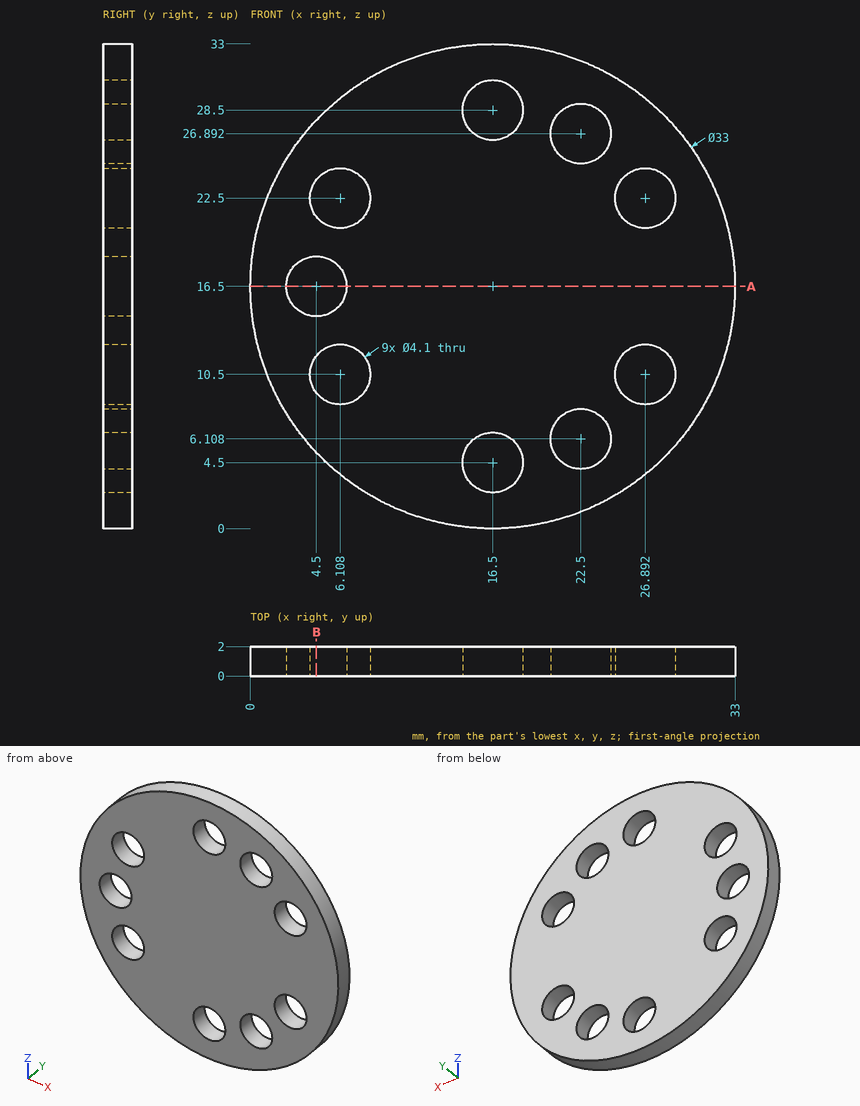
Geometry check sheet. Reference: drawing and pictorial views, mm from the part's lowest x, y, z. Round coordinates to 2 decimals unless told otherwise and drop trailing zeros. Order: outer loops, then holes, each group sorted by start corner. A loop starts at its lowest first (then second) coordinate and runs counter-clockwise, first axis right, second up. Notation, with made-up numbers: (13, 63.5) - (68, 63.5) arc R6 ccw to (68, 67.5) - close; hole circle Ø7 at (74, 49). An arc over 180 degrees is marked (long way). One line per question, with ' | ' between items. Start each with the question number.
(1) Sectioned sample at A-A on z = 16.5. Record the cut outline in (x, y).
(2) Sectioned sample at B-B on x = 4.5. Count the separate pieces of the cut face and the enclosed holes in it, and give its area (3 significant figures).
(3) Thickness scan on L1, parallel to X at y = 1.05, z = 16.5; L2, parallel to X at y = 1.2, z = 10 (1 decimal); L3, parallel to X at y = 0.8, z = 22.5. Record the ranges inside material, lowest first. Write a range as [from, to].
(4) Depth check by flat-ended pin: pin 1 Ø3.5 at (x, z) = (26.89, 10.5) entering from +Y; pin 2 Ø6 at (x, z) = (11, 6.5) entering from -Y. Enter the tip coordinate at first touch or a pass-through.
Conclusion:
1) outline: (0, 0) - (2.45, 0) - (2.45, 2) - (0, 2) - close; (6.55, 0) - (33, 0) - (33, 2) - (6.55, 2) - close
2) separate pieces: 4 | enclosed holes: 0 | area: 26.9 mm2
3) L1: x = [0, 2.45], [6.55, 33] | L2: x = [1.3, 4.1], [8.1, 24.9], [28.9, 31.7] | L3: x = [1.13, 4.06], [8.16, 24.84], [28.94, 31.87]
4) pin 1: passes through | pin 2: stops at y = 0
